Input: dimensioned drawing with shaded views. Units: mm. Origin: part minimum x, y, z. Coordinates: 2 decimals unless noted, no trailing zeros. Order: outer loops, then holes, each group sorted by start corner. A loop starts at its lowest first (then second) coordinate and runs counter-clockwise, first axis right, second up. Notation, with made-up numbers: (61, 31.5) - (96, 31.5) arc R11 ccw to (96, 47.5) - close; hole circle Ø1 at (79, 14.5). An arc over 180 degrees is marked (long way). Answer as CSV lines item,"result". Start each with the question number.
Item 1: Section B-B (y = 2.5). Output: boundary loops of the cut face in (x, z).
Item 2: Section A-A (z = 77.5). Output: boundary loops of the cut face in (x, y), and give its area (3 significant figures).
Item 3: Material intervals for line 1 along Z through (x, y) = (12.5, 8.5); line 2 along X through (y, z) = (3.25, 77.5); line 3 along X through (y, z) = (17.25, 77.5), sorted ascending.
Item 4: Section C-C (x = 77.5). Output: boundary loops of the cut face in (y, z), and give its area (3 significant figures).
Item 5: First-contact query: pin 1 (7.5 mm diameter, centred on x = 80.5, z = 75.5, fed in from +Y). Flat tip, straight axial feed; report the tip coordinate or a pass-through.
Item 6: Draft query along X for the marked faces 1, 2 and 3. Return one class per face: +X half, -X half, draft (parallel to the pull), parting line (faces both ways), or undercut.
Item 7: Section D-D (z = 45). Output: boundary loops of the cut face in (x, y), and give its area (3 significant figures).
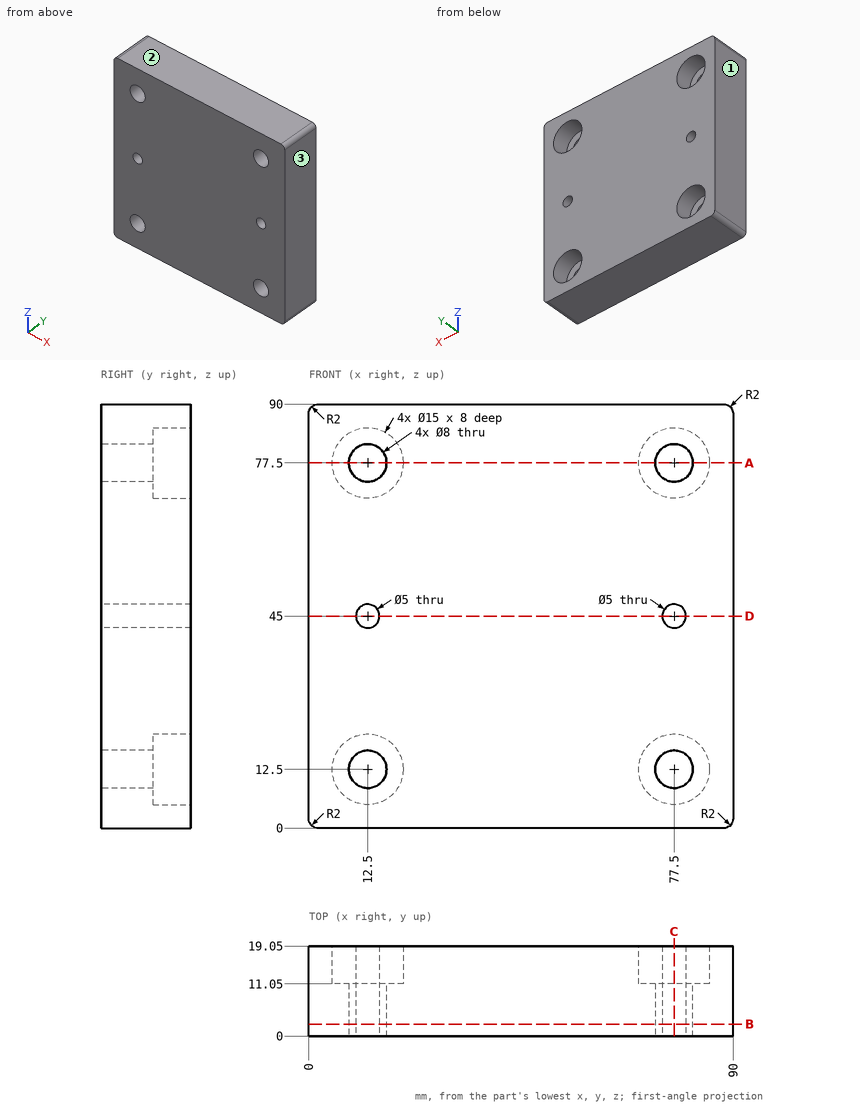
Determined:
1,outline,"(0, 2) arc R2 ccw to (2, 0) - (88, 0) arc R2 ccw to (90, 2) - (90, 88) arc R2 ccw to (88, 90) - (2, 90) arc R2 ccw to (0, 88) - close; hole circle Ø8 at (12.5, 12.5); hole circle Ø8 at (12.5, 77.5); hole circle Ø5 at (12.5, 45); hole circle Ø8 at (77.5, 12.5); hole circle Ø8 at (77.5, 77.5); hole circle Ø5 at (77.5, 45)"
2,outline,"(0, 0) - (8.5, 0) - (8.5, 11.05) - (5, 11.05) - (5, 19.05) - (0, 19.05) - close; (16.5, 0) - (73.5, 0) - (73.5, 11.05) - (70, 11.05) - (70, 19.05) - (20, 19.05) - (20, 11.05) - (16.5, 11.05) - close; (81.5, 0) - (90, 0) - (90, 19.05) - (85, 19.05) - (85, 11.05) - (81.5, 11.05) - close"
2,area,"1,300 mm^2"
3,line 1,"z = 0 to 8.5, 16.5 to 42.5, 47.5 to 73.5, 81.5 to 90"
3,line 2,"x = 0 to 8.5, 16.5 to 73.5, 81.5 to 90"
3,line 3,"x = 0 to 5, 20 to 70, 85 to 90"
4,outline,"(0, 0) - (19.05, 0) - (19.05, 5) - (11.05, 5) - (11.05, 8.5) - (0, 8.5) - close; (0, 16.5) - (11.05, 16.5) - (11.05, 20) - (19.05, 20) - (19.05, 42.5) - (0, 42.5) - close; (0, 47.5) - (19.05, 47.5) - (19.05, 70) - (11.05, 70) - (11.05, 73.5) - (0, 73.5) - close; (0, 81.5) - (11.05, 81.5) - (11.05, 85) - (19.05, 85) - (19.05, 90) - (0, 90) - close"
4,area,"1,200 mm^2"
5,pin 1,"stops at y = 11.05"
6,face 1,"-X half"
6,face 2,"draft"
6,face 3,"+X half"
7,outline,"(0, 0) - (10, 0) - (10, 19.05) - (0, 19.05) - close; (15, 0) - (75, 0) - (75, 19.05) - (15, 19.05) - close; (80, 0) - (90, 0) - (90, 19.05) - (80, 19.05) - close"
7,area,"1,520 mm^2"
